Check sheet for the modelled part. Datum: model origin and axes. Units: mm. Face numbers are marked on the shaded views. A direction names the side the tool comes from. Coordinates: 2 decimals unless noted, no trailing zeros. Order: outer loops, then holes, each group sorted by start corner. A loop starts at its lowest first (then second) coordinate and runs counter-clockwise, first axis right, second up. Notation, with made-up numbers: M 8,62.25 L 24,62.25 A32 ccw 24,92.25 Z; hole C 16,11.5 d7. An arc over 180 degrees is marked long. Answer in a Markdown table with one row per item. Add a question column.
from build123d import *

# Parameters (mm, degrees)
F1_DEPTH = 63.5
F0_W     = 25.348484695
F0_H     = 19.05
F2_DEPTH = 25.4
F3_DEPTH = 12.7
F5_R     = 5.08


with BuildPart() as f1:
    # F0 (on Front) → F1 (new body, symmetric)
    with BuildSketch(Plane.XZ):
        Polygon((22.225, 9.525), (-41.275, 9.525), (-41.275, -9.525), (41.275, -9.525), (41.275, 9.525), align=None)
    extrude(amount=F1_DEPTH, both=True)

    # F0 (on Front) → F2 (join, symmetric)
    with BuildSketch(Plane.XZ):
        with BuildLine():
            Line((22.225, 27.0002), (22.225, 9.525))
            Line((22.225, 9.525), (41.275, 9.525))
            Line((41.275, 9.525), (41.275, 27.0002))
            ThreePointArc((41.275, 27.0002), (45.9246798487, 38.2255201513), (57.15, 42.8752))
            Line((57.15, 42.8752), (60.376515305, 42.8752))
            Line((60.376515305, 42.8752), (60.376515305, 61.9252))
            Line((60.376515305, 61.9252), (57.15, 61.9252))
            ThreePointArc((57.15, 61.9252), (32.4542956671, 51.6959043329), (22.225, 27.0002))
        make_face()
        with Locations((73.0507576525, 52.4002)):
            Rectangle(F0_W, F0_H)
    extrude(amount=F2_DEPTH, both=True)

    # F0 (on Front) → F3 (join, symmetric)
    with BuildSketch(Plane.XZ):
        with BuildLine():
            add(Edge.make_bspline(
                [(-41.275, 9.525), (-27.2249449044, 51.4013841748), (17.066590488, 64.118757844), (57.15, 61.9252)],
                knots=[0, 0, 0, 0, 111.5045361635, 111.5045361635, 111.5045361635, 111.5045361635], degree=3))
            Line((-41.275, 9.525), (22.225, 9.525))
            Line((22.225, 9.525), (22.225, 27.0002))
            ThreePointArc((22.225, 27.0002), (32.4542956671, 51.6959043329), (57.15, 61.9252))
        make_face()
    extrude(amount=F3_DEPTH, both=True)

    # F0 (on Front) → F4 (revolve)
    with BuildSketch(Plane.XZ):
        Polygon((111.176515305, 66.675), (85.776515305, 66.675), (85.725, 38.1), (111.176515305, 38.1), align=None)
    revolve(axis=Axis((85.7507576525, 0, 52.3875), (-0.0018028074, 0, -0.9999983749)))

    # F5
    f5_edges = [f1.edges().sort_by_distance(p)[0] for p in [
        (-41.275, -63.5, 0),
        (41.275, -63.5, 0),
        (41.275, 63.5, 0),
        (-41.275, 63.5, 0),
    ]]
    fillet(f5_edges, radius=F5_R)


solid = f1.part
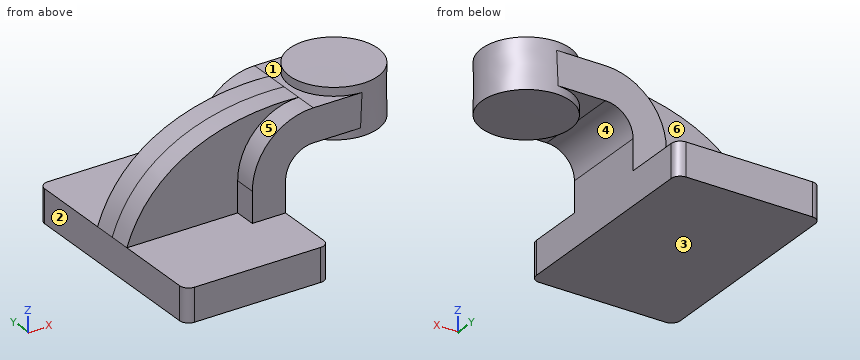
1. Set-up check for the marked faces 5 and 6: record each of +Z, -Z, +X, -X, +Y, -Y from which the full face is reachable in a straight line by a thin tool's end or side.
2. Section check A-A on z = -2.5. Enter the section's corners in (x, y) (3 decimals), then the cut area to 3 significant figures.
3. Go/stop test with flat-tipped pins: pin 1 Ø10 at (y, z) = (-18, 21.5) entering from -X (3 decimals); pin 2 Ø8 at (x, y) = (71.5, 10.5) entering from -Z; pin 3 Ø15.5 at (x, z) = (51.5, 34) entering from -Y. Record where each tip stops, or that it passes through.
4. Section check B-B on y = -41.5. Enter the section's corners in (x, z) (3 decimals), then the cut area to 3 significant figures.
5. Scan lines: line 1 (Z direction, x = 11, y = 54) (3 decimals); line 2 (Z direction, x = 82.5, y = 4.5); line 3 (X direction, y = -18, z = 11) (3 decimals). Record each from-to range of solid material in increasing order.
6. Release check for a two-part mould opening along X. For the marked faces 1, 2, 3 and 4 record: released by +X, released by -X, zero draft, split by the parting line, or undercut.
Result sheet:
| question | item | result |
|---|---|---|
| 1 | face 5 | +Z, -X, -Y |
| 1 | face 6 | +Z, -X, +Y |
| 2 | outline | M -41.275,-58.42 A5.08 ccw -36.195,-63.5 L 36.195,-63.5 A5.08 ccw 41.275,-58.42 L 41.275,58.42 A5.08 ccw 36.195,63.5 L -36.195,63.5 A5.08 ccw -41.275,58.42 Z |
| 2 | area | 10,500 mm^2 |
| 3 | pin 1 | x = 22.225 |
| 3 | pin 2 | z = 38.14 |
| 3 | pin 3 | y = -25.4 |
| 4 | outline | M -41.275,-9.525 L 41.275,-9.525 L 41.275,9.525 L -41.275,9.525 Z |
| 4 | area | 1,570 mm^2 |
| 5 | line 1 | -9.525 to 9.525 |
| 5 | line 2 | 38.12 to 66.69 |
| 5 | line 3 | 22.225 to 41.275 |
| 6 | face 1 | undercut |
| 6 | face 2 | released by -X |
| 6 | face 3 | zero draft |
| 6 | face 4 | undercut |
